```python
from build123d import *

# Parameters (mm, degrees)
F2_DEPTH = 9
F3_DEPTH = 7


with BuildPart() as f2:
    # F1 (on Front) → F2 (new body)
    with BuildSketch(Plane.XZ):
        Polygon((-75.443379581, 10.1466504857), (-74.6737569571, 8.2548242062), (-49.936760217, 8.2548242062), (-5.3362287581, -39.0802323818), (-3.9785234258, -37.1320582926), (-48.8134101033, 10.1466504857), align=None)
    extrude(amount=F2_DEPTH)



with BuildPart() as f2b:
    # F1 (on Front) → F2, piece 2 (new body)
    with BuildSketch(Plane.XZ):
        Polygon((75.443379581, 10.1466504857), (48.8134101033, 10.1466504857), (3.9785234258, -37.1320582926), (5.3362287581, -39.0802323818), (49.936760217, 8.2548242062), (74.6737569571, 8.2548242062), align=None)
    extrude(amount=F2_DEPTH)


with BuildPart() as f2_1:
    add(f2.part)

    add(f2b.part)  # F3 merges F2b
    # F0 (on Front) → F3 (join)
    with BuildSketch(Plane.XZ):
        Polygon((-74.166752398, 7.2823497467), (-71.30458951, 1.5580287436), (-47.5895479321, 1.5580287436), (-13.5767729953, -33.0098701724), (0, -10.5720795691), (13.5767729953, -33.0098701724), (47.5895479321, 1.5580287436), (71.30458951, 1.5580287436), (74.166752398, 7.2823497467), (46.3629066944, 7.2823497467), (15.8331952989, -24.7465875), (4.8833945766, 4.0167045015), (-2.0373270524, 4.0167045015), (-8.6096497253, -1.7130117631), (-3.9756768383, -7.0284521207), (-15.8331952989, -24.7465875), (-46.3629066944, 7.2823497467), align=None)
        Polygon((13.5767729953, -36.478985101), (0, -13.3794201538), (-13.5767729953, -36.478985101), (-49.4699440897, 0), (-70.081859827, 0), (-65.8173263073, -8.4041291848), (-54.0898554027, -8.4041291848), (-13.5767729953, -50.3387264907), (-6.7883864976, -41.0989001393), (-4.3703924554, -37.8077137762), (0, -31.8590737879), (13.5767729953, -50.3387264907), (54.0898554027, -8.4041291848), (65.8173263073, -8.4041291848), (70.081859827, 0), (49.4699440897, 0), align=None)
    extrude(amount=F3_DEPTH)


solid = f2_1.part
```
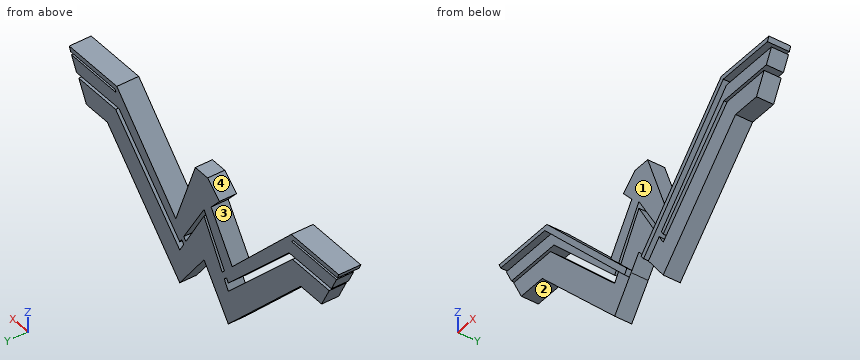
The listing builds one solid part. Answer for the finished solid, in the listing's coordinates (mm). Face numbers are marked on the shaded views. A direction names the side the tool comes from. Give positions to 0.01 mm unless a question says otherwise; leave off trailing zeros. Loops run counter-clockwise (first coordinate to the right, second up) from the corner with the lowest first, then second, coordinate; pieces in that order, holes last. Notation, with made-up numbers: M 89,21.25 L 109,21.25 A22 ccw 109,33.25 Z; hole C 21.25,19.5 d1. An arc over 180 degrees is marked long. One line per item, written item: value.
1. Each of these flat-tipped pins is pushed along its axis until it touches: P1, Ø3, axis at y = -1.5, z = -30.5, coming from the -X side; P2, Ø3.5, axis at x = 58.5, y = -5, coming from the -Z side; P3, Ø9.5, axis at x = -6.5, z = -20, coming from the -Y side. Where does it stop, or does it pass through?
Found:
P1: x = -34.19
P2: z = -8.4
P3: y = -7
2. Find the intervals of material crossed by probe 1 along Z at (x, y) = (-57.5, -4.5); probe 2 along X at (y, z) = (-1, 0.5); probe 3 along Z at (x, y) = (67, -5.5), in increasing order.
Found:
probe 1: -8.4 to 0, 1.56 to 7.28, 8.25 to 10.15
probe 2: -46.55 to -39.67, -6.07 to 6.22, 39.67 to 46.55
probe 3: -6.07 to 0, 1.56 to 7.28, 8.25 to 10.15
3. Section D-D on z = -44 is taken. Determine the outline of the cut face in (x, y).
Found:
outline: M -19.7,-7 L -8.92,-7 L -8.92,0 L -19.7,0 Z; M 8.92,-7 L 19.7,-7 L 19.7,0 L 8.92,0 Z
4. Section A-A on x = -59 is taken. Determine the outline of the cut face in (y, z).
Found:
outline: M -9,8.25 L 0,8.25 L 0,10.15 L -9,10.15 Z; M -7,-8.4 L 0,-8.4 L 0,0 L -7,0 Z; M -7,1.56 L 0,1.56 L 0,7.28 L -7,7.28 Z
5. Section C-C on z = -5.5 is taken. Determine the outline of the cut face in (x, y), plus the area to 3 significant figures.
Found:
outline: M -67.29,-7 L -44.06,-7 L -44.06,0 L -67.29,0 Z; M -40.64,-7 L -36.98,-7 L -36.98,-9 L -33.98,-9 L -33.98,0 L -40.64,0 Z; M -5.31,-7 L 8.51,-7 L 8.51,0 L -5.31,0 Z; M 33.98,-9 L 36.98,-9 L 36.98,-7 L 40.64,-7 L 40.64,0 L 33.98,0 Z; M 44.06,-7 L 67.29,-7 L 67.29,0 L 44.06,0 Z
area: 527 mm^2
6. For the marked faces 1, 2, 3 and 4, determine the directions among +Z, -Z, +X, -X, +Y, -Y from which every point of the face is accessible in a straight line to the end or side of a thin tool.
Found:
face 1: +Z, -Y
face 2: -Z, -X, +Y, -Y
face 3: +Y, -Y
face 4: +Z, +Y, -Y
7. Section B-B on x = -20 is taken. Determine the outline of the cut face in (y, z).
Found:
outline: M -9,-23.52 L -7,-23.52 L -7,-26.48 L 0,-26.48 L 0,-20.24 L -9,-20.24 Z; M -7,-43.69 L 0,-43.69 L 0,-29.95 L -7,-29.95 Z
